Could you check a few things on this model? Use its own coordinates, in mm. A direction names the side the tool comes from. Coordinates: 2 decimals unless noted, no trailing zeros. Order: outer loops, then holes, each group sorted by start corner. A loop starts at its lowest first (then second) coordinate and runs counter-clockwise, first axis right, second up. Notation, with made-up numbers: M 26,8.25 L 45,8.25 A29 cw 45,41.25 Z; hole C 40,15 d7. An arc over 180 degrees is marked long. Put each result on its own line as item: value. Start each with the question number.
```python
from build123d import *

# Parameters (mm, degrees)
SKETCH1_R           = 5
BOSS_EXTRUDE1_DEPTH = 70
SKETCH2_R           = 4.5
BOSS_EXTRUDE2_DEPTH = 6
SKETCH3_R           = 5
CUT_EXTRUDE2_DEPTH  = 0.88667719
SKETCH4_R           = 4
BOSS_EXTRUDE3_DEPTH = 7
BOSS_EXTRUDE4_START = 65
SKETCH5_R           = 5
BOSS_EXTRUDE4_DEPTH = 65


with BuildPart() as part:
    # Sketch1 → Boss-Extrude1 (new body)
    with BuildSketch(Plane.XY):
        Circle(SKETCH1_R)
    extrude(amount=BOSS_EXTRUDE1_DEPTH)

    # Sketch2 → Boss-Extrude2 (add)
    with BuildSketch(Plane(origin=(0, 0, 0), x_dir=(1, 0, 0), z_dir=(0, 1, 0))):
        with Locations(Location((0, -5.386677191, 0), (0, 0, 90))):
            Circle(SKETCH2_R)
    extrude(amount=BOSS_EXTRUDE2_DEPTH)

    # Sketch3 → Cut-Extrude2 (cut)
    with BuildSketch(Plane(origin=(0, 0, 0), x_dir=(-1, 0, 0), z_dir=(0, 0, -1))):
        with Locations(Location((0, 0, 0), (0, 0, 90))):
            Circle(SKETCH3_R)
    extrude(amount=-CUT_EXTRUDE2_DEPTH, mode=Mode.SUBTRACT)

    # Sketch4 → Boss-Extrude3 (add)
    with BuildSketch(Plane(origin=(0, 6, 0), x_dir=(1, 0, 0), z_dir=(0, 1, 0))):
        with Locations(Location((0, -5.386677191, 0), (0, 0, 270))):
            Circle(SKETCH4_R)
    extrude(amount=BOSS_EXTRUDE3_DEPTH)

    # Sketch5 → Boss-Extrude4 (add)
    with BuildSketch(Plane(origin=(0, 0, 0.88667719), x_dir=(-1, 0, 0), z_dir=(0, 0, -1)).offset(BOSS_EXTRUDE4_START)):
        Circle(SKETCH5_R)
    extrude(amount=-BOSS_EXTRUDE4_DEPTH)


solid = part.part
```
Item 1: For faces 1 (the cylindrical face through (-3.794, 4.487, 2.968)), 2 (the flat face through (0, 0, -64.113)), which set-ups out of +Z, -Z, +X, -X, +Y, -Y let a thin tool reach every point of the face, with its end or its side?
Item 2: If we section it at A-A on z = 4.5: Write out the boundary of the cut face in (x, y).
Item 3: For pin 1 Ø5 at (x, z) = (-3.5, 46) entering from +Y; pin 2 Ø10 at (y, z) = (7, 14) entering from -X, each with a flat end and sliding along its axis, tell me the tip position at first contact or that it passes through.
Item 4: If we section it at B-B on x = 0: Write out the boundary of the cut face in (y, z).
Item 5: If we section it at D-D on z = 60: Write out the boundary of the cut face in (x, y).
Item 6: If we section it at C-C on y = -2.75: Write out the boundary of the cut face in (x, z), then the cut area to 3 significant figures.
Item 7: I need wall thicknesses on probe 1 along X at (y, z) = (3, 27.5); probe 2 along Y at (x, z) = (0.75, 0); probe 3 along X at (y, z) = (1.5, 1). Which ranges of each line are inside material? Lowest first, please.
Geometry check:
1. face 1: +Y
1. face 2: -Z, +X, -X, +Y, -Y
2. outline: M -4.41,2.35 A5 ccw long 4.41,2.35 L 4.41,6 L 3.9,6 L 3.9,13 L -3.9,13 L -3.9,6 L -4.41,6 Z
3. pin 1: stops at y = 4.9
3. pin 2: stops at x = -4.58
4. outline: M -5,-64.11 L 5,-64.11 L 5,0.89 L 6,0.89 L 6,1.39 L 13,1.39 L 13,9.39 L 6,9.39 L 6,9.89 L 5,9.89 L 5,70 L -5,70 Z
5. outline: C 0,0 d10
6. outline: M -4.18,-64.11 L 4.18,-64.11 L 4.18,70 L -4.18,70 Z
6. area: 1,120 mm²
7. probe 1: x = -4 to 4
7. probe 2: y = -4.94 to 4.94
7. probe 3: x = -4.77 to 4.77
